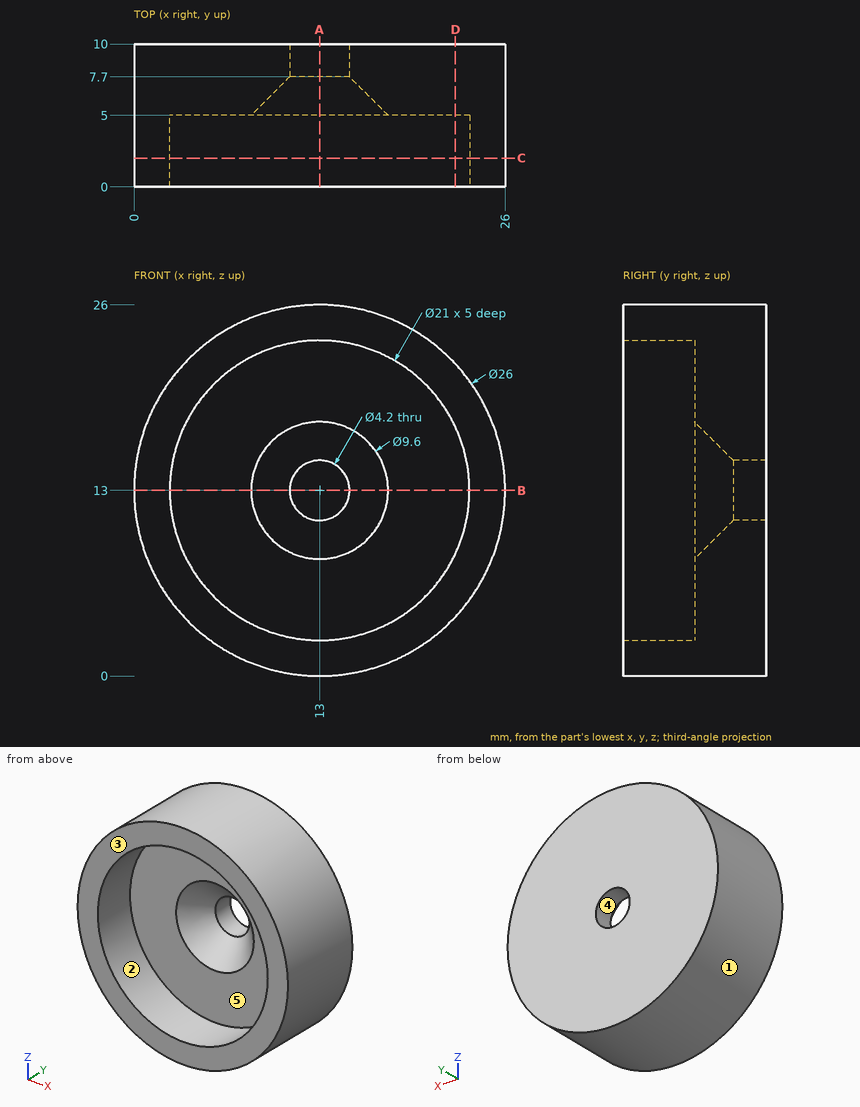
Here's the drawing with two shaded views (mm, measured from the low corner). I have some questions. A direction names the side the tool comes from. Coordinates: 2 decimals unless noted, no trailing zeros. Write each loop counter-clockwise with the first axis right and the second up, starting at its lowest first coordinate (ties: lowest second). Pieces come first, ordered by that corner, then holes. Notation, with made-up numbers: (-40, -20.5) -> (18, -20.5) arc R24 cw to (18, -10.5) -> close; hole circle Ø6 at (27.5, 25). An arc over 180 degrees is marked (long way). One line per question, with ' | ' between items. Start each with the question number.
1. If we section it at B-B (z = 13): Please give me the cut outline in (x, y).
2. If we section it at A-A (x = 13): Please give me the cut outline in (y, z), and give its area (3 significant figures).
3. Thinking about a two-plate mould opening in Z: for the marked faces 1, 2 and 3, which applies, pulls with the +Z half, pulls with the -Z half, needs draft (parallel to the pull), parting line crosses it, or undercut?
4. If we section it at D-D (x = 22.5): Please give me the cut outline in (y, z), and give its area (3 significant figures).
5. If we section it at C-C (y = 2): Please give me the cut outline in (x, z), and give its area (3 significant figures).
6. For the marked faces 4 and 5, which set-ups out of +Z, -Z, +X, -X, +Y, -Y let a thin tool reach every point of the face, with its end or its side?
7. Please list where these lines run through material, in increasing order: line 1 along Z through (x, y) = (13, 3.5); line 2 along Z through (x, y) = (13, 8.8); line 3 along Y through (x, z) = (16.5, 18).
8. Will these pins go through, and if not, where does the flat tip stop? P1, Ø8, axis at x = 13, z = 3, coming from the -Y side; P2, Ø6.5, axis at x = 13.5, z = 10, coming from the -Y side; P3, Ø1, axis at x = 4.5, y = 3, coming from the -Z side; P4, Ø1, axis at x = 11, z = 16, coming from the -Y side.
Return value:
1) outline: (0, 0) -> (2.5, 0) -> (2.5, 5) -> (8.2, 5) -> (10.9, 7.7) -> (10.9, 10) -> (0, 10) -> close; (15.1, 7.7) -> (17.8, 5) -> (23.5, 5) -> (23.5, 0) -> (26, 0) -> (26, 10) -> (15.1, 10) -> close
2) outline: (0, 0) -> (10, 0) -> (10, 10.9) -> (7.7, 10.9) -> (5, 8.2) -> (5, 2.5) -> (0, 2.5) -> close; (0, 23.5) -> (5, 23.5) -> (5, 17.8) -> (7.7, 15.1) -> (10, 15.1) -> (10, 26) -> (0, 26) -> close | area: 127 mm²
3) face 1: parting line crosses it | face 2: undercut | face 3: needs draft
4) outline: (0, 4.13) -> (10, 4.13) -> (10, 21.87) -> (0, 21.87) -> (0, 17.47) -> (5, 17.47) -> (5, 8.53) -> (0, 8.53) -> close | area: 133 mm²
5) outline: circle Ø26 at (13, 13); hole circle Ø21 at (13, 13) | area: 185 mm²
6) face 4: +Y, -Y | face 5: -Y
7) line 1: z = 0 to 2.5, 23.5 to 26 | line 2: z = 0 to 10.9, 15.1 to 26 | line 3: y = 5 to 10
8) P1: stops at y = 0 | P2: stops at y = 5 | P3: stops at z = 2.75 | P4: stops at y = 5.69
